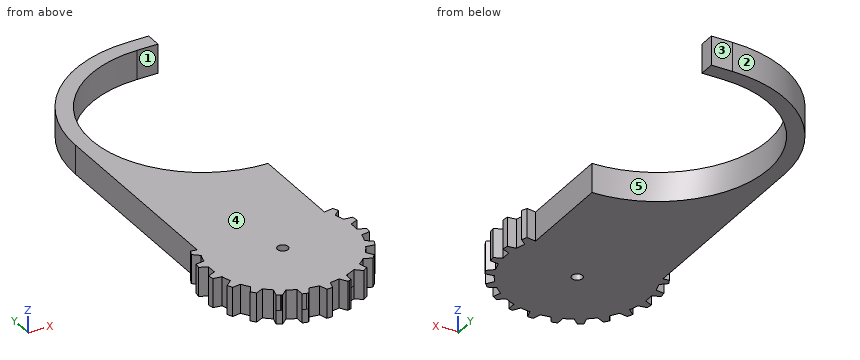
from build123d import *

# Parameters (mm, degrees)
BOSS_EXTRUDE1_DEPTH = 3
SKETCH3_W           = 3
SKETCH3_H           = 3
BOSS_EXTRUDE2_DEPTH = 4
BOSS_EXTRUDE3_START = 2.5
BOSS_EXTRUDE3_DEPTH = 2.5
CUT_EXTRUDE1_REACH  = 68.382
SKETCH5_R           = 1


with BuildPart() as part:
    # Sketch1 → Boss-Extrude1 (new body)
    with BuildSketch(Plane.XY):
        with BuildLine():
            ThreePointArc((0, -21), (-21, 0), (0, 21))
            Line((0, 21), (0, 24))
            ThreePointArc((0, 24), (-16.970562748, 16.970562748), (-24, 0))
            Line((-24, 0), (-24, -38.951706039))
            Line((-24, -38.951706039), (-25.1251405, -38.782264509))
            Line((-25.1251405, -38.782264509), (-25.583788433, -39.786563393))
            Line((-25.583788433, -39.786563393), (-24.347066616, -40.843822809))
            ThreePointArc((-24.347066616, -40.843822809), (-24.638511224, -41.723497067), (-24.868920228, -42.621092996))
            Line((-24.868920228, -42.621092996), (-26.480914421, -42.841893921))
            Line((-26.480914421, -42.841893921), (-26.638040197, -43.934727699))
            Line((-26.638040197, -43.934727699), (-25.153549904, -44.60073588))
            ThreePointArc((-25.153549904, -44.60073588), (-25.18535608, -45.526886585), (-25.153549904, -46.453037289))
            Line((-25.153549904, -46.453037289), (-26.638040197, -47.119045471))
            Line((-26.638040197, -47.119045471), (-26.48091442, -48.211879248))
            Line((-26.48091442, -48.211879248), (-24.868920228, -48.432680173))
            ThreePointArc((-24.868920228, -48.432680173), (-24.638511224, -49.330276102), (-24.347066616, -50.20995036))
            Line((-24.347066616, -50.20995036), (-25.583788433, -51.267209776))
            Line((-25.583788433, -51.267209776), (-25.1251405, -52.271508661))
            Line((-25.1251405, -52.271508661), (-23.516236589, -52.029214351))
            ThreePointArc((-23.516236589, -52.029214351), (-23.042278774, -52.82553762), (-22.514806841, -53.587469455))
            Line((-22.514806841, -53.587469455), (-23.403568337, -54.950327236))
            Line((-23.403568337, -54.950327236), (-22.680555175, -55.784728904))
            Line((-22.680555175, -55.784728904), (-21.205085373, -55.098968604))
            ThreePointArc((-21.205085373, -55.098968604), (-20.525975989, -55.729505838), (-19.805209372, -56.311968064))
            Line((-19.805209372, -56.311968064), (-20.274008375, -57.870013577))
            Line((-20.274008375, -57.870013577), (-19.674605945, -58.255226128))
            Line((-19.674605945, -58.255226128), (-19.50868057, -58.361859893))
            Line((-19.50868057, -58.361859893), (-19.345204211, -58.466919769))
            Line((-19.345204211, -58.466919769), (-18.122702306, -57.393249699))
            ThreePointArc((-18.122702306, -57.393249699), (-17.293458756, -57.806918522), (-16.437789679, -58.162723513))
            Line((-16.437789679, -58.162723513), (-16.448646882, -59.789733177))
            Line((-16.448646882, -59.789733177), (-15.747386057, -59.995641934))
            Line((-15.747386057, -59.995641934), (-15.389297906, -60.100786102))
            Line((-15.389297906, -60.100786102), (-14.518803732, -58.726188627))
            ThreePointArc((-14.518803732, -58.726188627), (-13.606606397, -58.88947605), (-12.68535608, -58.989798602))
            Line((-12.68535608, -58.989798602), (-12.237391898, -60.553961771))
            Line((-12.237391898, -60.553961771), (-11.133320263, -60.553961771))
            Line((-11.133320263, -60.553961771), (-10.68535608, -58.989798602))
            ThreePointArc((-10.68535608, -58.989798602), (-9.764105764, -58.88947605), (-8.851908429, -58.726188627))
            Line((-8.851908429, -58.726188627), (-7.986392322, -60.092925234))
            Line((-7.986392322, -60.092925234), (-7.623326104, -59.995641934))
            Line((-7.623326104, -59.995641934), (-7.262677826, -59.889746045))
            Line((-7.262677826, -59.889746045), (-7.234972221, -58.272241954))
            ThreePointArc((-7.234972221, -58.272241954), (-7.083621531, -58.21838134), (-6.932922481, -58.162723513))
            ThreePointArc((-6.932922481, -58.162723513), (-6.077253405, -57.806918522), (-5.248009855, -57.393249699))
            Line((-5.248009855, -57.393249699), (-4.025507949, -58.466919769))
            Line((-4.025507949, -58.466919769), (-3.096703786, -57.870013577))
            Line((-3.096703786, -57.870013577), (-3.565502789, -56.311968064))
            ThreePointArc((-3.565502789, -56.311968064), (-2.844736172, -55.729505838), (-2.165626787, -55.098968604))
            Line((-2.165626787, -55.098968604), (-0.690156985, -55.784728904))
            Line((-0.690156985, -55.784728904), (0.032856176, -54.950327236))
            Line((0.032856176, -54.950327236), (-0.855905319, -53.587469455))
            ThreePointArc((-0.855905319, -53.587469455), (-0.328433387, -52.82553762), (0.145524429, -52.029214351))
            Line((0.145524429, -52.029214351), (1.754428339, -52.27150866))
            Line((1.754428339, -52.27150866), (2.213076272, -51.267209776))
            Line((2.213076272, -51.267209776), (0.976354455, -50.20995036))
            ThreePointArc((0.976354455, -50.20995036), (1.267799063, -49.330276102), (1.498208067, -48.432680173))
            Line((1.498208067, -48.432680173), (3.11020226, -48.211879248))
            Line((3.11020226, -48.211879248), (3.267328036, -47.11904547))
            Line((3.267328036, -47.11904547), (1.782837743, -46.453037289))
            ThreePointArc((1.782837743, -46.453037289), (1.81464392, -45.526886584), (1.782837743, -44.60073588))
            Line((1.782837743, -44.60073588), (3.267328036, -43.934727698))
            Line((3.267328036, -43.934727698), (3.11020226, -42.84189392))
            Line((3.11020226, -42.84189392), (1.498208067, -42.621092996))
            ThreePointArc((1.498208067, -42.621092996), (1.267799063, -41.723497067), (0.976354455, -40.843822809))
            Line((0.976354455, -40.843822809), (2.213076272, -39.786563393))
            Line((2.213076272, -39.786563393), (1.754428339, -38.782264508))
            Line((1.754428339, -38.782264508), (0, -39.046474198))
            Line((0, -39.046474198), (0, -36.153828735))
            Line((0, -36.153828735), (0, -36.065527885))
            Line((0, -36.065527885), (0, -21))
        make_face()
    extrude(amount=BOSS_EXTRUDE1_DEPTH)

    # Sketch3 → Boss-Extrude2 (add)
    with BuildSketch(Plane(origin=(0, 0, 0), x_dir=(0, 0, -1), z_dir=(1, 0, 0))):
        with Locations((-1.5, 22.5)):
            Rectangle(SKETCH3_W, SKETCH3_H)
    extrude(amount=BOSS_EXTRUDE2_DEPTH)

    # Sketch4 → Boss-Extrude3 (add)
    with BuildSketch(Plane(origin=(0, 0, 0), x_dir=(-1, 0, 0), z_dir=(0, 0, -1)).offset(BOSS_EXTRUDE3_START)):
        with BuildLine():
            Line((-1.498208067, -42.621092996), (-3.11020226, -42.84189392))
            Line((-3.11020226, -42.84189392), (-3.267328036, -43.934727698))
            Line((-3.267328036, -43.934727698), (-1.782837743, -44.60073588))
            ThreePointArc((-1.782837743, -44.60073588), (-1.81464392, -45.526886584), (-1.782837743, -46.453037289))
            Line((-1.782837743, -46.453037289), (-3.267328036, -47.11904547))
            Line((-3.267328036, -47.11904547), (-3.11020226, -48.211879248))
            Line((-3.11020226, -48.211879248), (-1.498208067, -48.432680173))
            ThreePointArc((-1.498208067, -48.432680173), (-1.267799063, -49.330276102), (-0.976354455, -50.20995036))
            Line((-0.976354455, -50.20995036), (-2.213076272, -51.267209776))
            Line((-2.213076272, -51.267209776), (-1.754428339, -52.27150866))
            Line((-1.754428339, -52.27150866), (-0.145524429, -52.029214351))
            ThreePointArc((-0.145524429, -52.029214351), (0.328433387, -52.82553762), (0.855905319, -53.587469455))
            Line((0.855905319, -53.587469455), (-0.032856176, -54.950327236))
            Line((-0.032856176, -54.950327236), (0.690156985, -55.784728904))
            Line((0.690156985, -55.784728904), (2.165626787, -55.098968604))
            ThreePointArc((2.165626787, -55.098968604), (2.844736172, -55.729505838), (3.565502789, -56.311968064))
            Line((3.565502789, -56.311968064), (3.096703786, -57.870013577))
            Line((3.096703786, -57.870013577), (4.025507949, -58.466919769))
            Line((4.025507949, -58.466919769), (5.248009855, -57.393249699))
            ThreePointArc((5.248009855, -57.393249699), (6.223779069, -57.872783739), (7.234972221, -58.272241954))
            Line((7.234972221, -58.272241954), (7.262677826, -59.889746045))
            Line((7.262677826, -59.889746045), (7.623326104, -59.995641934))
            Line((7.623326104, -59.995641934), (7.986392322, -60.092925234))
            Line((7.986392322, -60.092925234), (8.851908429, -58.726188627))
            ThreePointArc((8.851908429, -58.726188627), (9.764105764, -58.88947605), (10.68535608, -58.989798602))
            Line((10.68535608, -58.989798602), (11.133320263, -60.553961771))
            Line((11.133320263, -60.553961771), (12.237391898, -60.553961771))
            Line((12.237391898, -60.553961771), (12.68535608, -58.989798602))
            ThreePointArc((12.68535608, -58.989798602), (13.606606397, -58.88947605), (14.518803732, -58.726188627))
            Line((14.518803732, -58.726188627), (15.389297906, -60.100786102))
            Line((15.389297906, -60.100786102), (16.448646882, -59.789733177))
            Line((16.448646882, -59.789733177), (16.437789679, -58.162723513))
            ThreePointArc((16.437789679, -58.162723513), (17.293458756, -57.806918522), (18.122702306, -57.393249699))
            Line((18.122702306, -57.393249699), (19.345204211, -58.466919769))
            Line((19.345204211, -58.466919769), (20.274008375, -57.870013577))
            Line((20.274008375, -57.870013577), (19.805209372, -56.311968064))
            ThreePointArc((19.805209372, -56.311968064), (20.525975989, -55.729505838), (21.205085373, -55.098968604))
            Line((21.205085373, -55.098968604), (22.680555175, -55.784728904))
            Line((22.680555175, -55.784728904), (23.403568337, -54.950327236))
            Line((23.403568337, -54.950327236), (22.514806841, -53.587469455))
            ThreePointArc((22.514806841, -53.587469455), (23.042278774, -52.82553762), (23.516236589, -52.029214351))
            Line((23.516236589, -52.029214351), (25.1251405, -52.271508661))
            Line((25.1251405, -52.271508661), (25.583788433, -51.267209776))
            Line((25.583788433, -51.267209776), (24.347066616, -50.20995036))
            ThreePointArc((24.347066616, -50.20995036), (24.638511224, -49.330276102), (24.868920228, -48.432680173))
            Line((24.868920228, -48.432680173), (26.48091442, -48.211879248))
            Line((26.48091442, -48.211879248), (26.638040197, -47.119045471))
            Line((26.638040197, -47.119045471), (25.153549904, -46.453037289))
            ThreePointArc((25.153549904, -46.453037289), (25.18535608, -45.526886585), (25.153549904, -44.60073588))
            Line((25.153549904, -44.60073588), (26.638040197, -43.934727699))
            Line((26.638040197, -43.934727699), (26.480914421, -42.841893921))
            Line((26.480914421, -42.841893921), (24.868920228, -42.621092996))
            ThreePointArc((24.868920228, -42.621092996), (24.638511224, -41.723497067), (24.347066616, -40.843822809))
            Line((24.347066616, -40.843822809), (25.583788433, -39.786563393))
            Line((25.583788433, -39.786563393), (25.1251405, -38.782264509))
            Line((25.1251405, -38.782264509), (24, -38.951706039))
            Line((24, -38.951706039), (24, 0))
            ThreePointArc((24, 0), (16.970562748, 16.970562748), (0, 24))
            Line((0, 24), (-4, 24))
            Line((-4, 24), (-4, 21))
            Line((-4, 21), (0, 21))
            ThreePointArc((0, 21), (21, 0), (0, -21))
            Line((0, -21), (0, -39.046474198))
            Line((0, -39.046474198), (-1.754428339, -38.782264508))
            Line((-1.754428339, -38.782264508), (-2.213076272, -39.786563393))
            Line((-2.213076272, -39.786563393), (-0.976354455, -40.843822809))
            ThreePointArc((-0.976354455, -40.843822809), (-1.267799063, -41.723497067), (-1.498208067, -42.621092996))
        make_face()
    extrude(amount=-BOSS_EXTRUDE3_DEPTH)

    # Sketch5 → Cut-Extrude1 (cut, up to next)
    with BuildSketch(Plane.XY.offset(3), mode=Mode.PRIVATE) as cut_extrude1_sk1:
        with Locations((-11.68535608, -45.526886584)):
            Circle(SKETCH5_R)
    cut_extrude1_tool1 = extrude(cut_extrude1_sk1.sketch, amount=-CUT_EXTRUDE1_REACH, mode=Mode.PRIVATE) & part.part
    add(cut_extrude1_tool1.solids().sort_by_distance((-11.685356, -45.526887, 3))[0], mode=Mode.SUBTRACT)


solid = part.part
Check sheet for the modelled part. Datum: model origin and axes. Units: mm. Face numbers are marked on the shaded views. A direction names the side the tool comes from. Give positions to 0.01 mm unless a question says otherwise; leave off trailing zeros. Loops run counter-clockwise (first coordinate to the right, second up) from the corner with the lowest first, then second, coordinate; pieces in that order, holes last. Notation, with made-up numbers: M -3,-7.75 L 52,-7.75 A30 ccw 52,22.25 Z; hole C 14.5,-24.75 d7. An arc over 180 degrees is marked long. Answer as a JSON object with one key per item and string values. Group by question number.
Q1. Release check for a two-part mould opening along Y. For the marked faces 3, 4 and 5 record: released by +Y, released by -Y, zero draft, split by the parting line, or undercut.
Q2. Access from +Z, -Z, +X, -X, +Y, -Y to the whole of each face (thin tool, end or side, straight path). Record for the marked faces 1 and 2.
Q3. Material ranges on line 1 along Y through (x, z) = (-3, -0.75); line 2 along Y through (x, z) = (-1, -0.95); line 3 along Y through (x, z) = (2, 1.8), recorded low to high. Write a range as [from, to].
Q4. Cross-section at A-A on y = -36. Record the cut outline in (x, z).
Q5. Cross-section at B-B on y = 9.5. Record the cut outline in (x, z), then the cut area to 3 significant figures.
Q6. Go/stop test with flat-tipped pins: P1, Ø1.6, axis at x = -11.69, y = -45.53, coming from the +Z side; P2, Ø1.6, axis at y = -25.5, z = 0.5, coming from the +X side; P3, Ø3, axis at y = -29, z = 1.5, coming from the -X side; P4, Ø3, axis at x = -16.5, z = 1, coming from the +Y side (3 decimals). Record where each tip stops, or that it passes through.
Evaluation:
{
 "1": {"face 3": "released by +Y", "face 4": "zero draft", "face 5": "undercut"},
 "2": {"face 1": "+Z, -Z, +X", "face 2": "+Z, -Z, -X, +Y"},
 "3": {"line 1": "y = [-55.86, -20.78], [20.78, 23.81]", "line 2": "y = [-55.64, -20.98], [20.98, 23.98]", "line 3": "y = [-51.73, -51.09], [-48.36, -46.55], [-44.5, -42.69], [-39.97, -39.32], [21, 24]"},
 "4": {"outline": "M -24,-2.5 L 0,-2.5 L 0,3 L -24,3 Z"},
 "5": {"outline": "M -22.04,-2.5 L -18.73,-2.5 L -18.73,3 L -22.04,3 Z", "area": "18.2 mm2"},
 "6": {"P1": "passes through", "P2": "stops at x = 0", "P3": "stops at x = -24", "P4": "stops at y = 18.735"}
}
